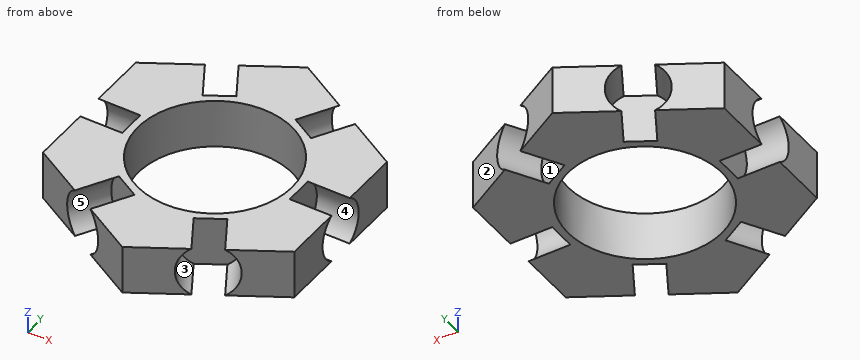
from build123d import *

# Parameters (mm, degrees)
SKETCH1_R           = 11
BOSS_EXTRUDE1_DEPTH = 3.5
SKETCH2_R           = 4.05
CUT_EXTRUDE3_DEPTH  = 6
CIRPATTERN1_COUNT   = 6


with BuildPart() as part:
    # Sketch1 → Boss-Extrude1 (new body, symmetric)
    with BuildSketch(Plane.XY):
        Polygon((18, -10.392304845), (18, 10.392304845), (0, 20.784609691), (-18, 10.392304845), (-18, -10.392304845), (0, -20.784609691), align=None)
        Circle(SKETCH1_R, mode=Mode.SUBTRACT)
    extrude(amount=BOSS_EXTRUDE1_DEPTH, both=True)

    # Sketch2 → Cut-Extrude3 (cut)
    with BuildSketch(Plane(origin=(-12.610372246, -13.50400788, 0), x_dir=(0.866025404, -0.5, 0), z_dir=(0.5, 0.866025404, 0))):
        with Locations((4.168898776, 0)):
            Circle(SKETCH2_R)
    cut_extrude3 = extrude(amount=CUT_EXTRUDE3_DEPTH, mode=Mode.SUBTRACT)

    # CirPattern1: Cut-Extrude3 ×6 about axis
    cirpattern1_axis = Axis((0, 0, 0), (0, 0, 1))
    for i in range(1, CIRPATTERN1_COUNT):
        add(cut_extrude3.rotate(cirpattern1_axis, i * 360 / CIRPATTERN1_COUNT), mode=Mode.SUBTRACT)


solid = part.part
CAD build for the part. Positions are in the model's coordinates, mm. Face numbers are marked on the shaded views. A direction names the side the tool comes from. Give positions to 0.01 mm unless a question says otherwise; leave off trailing zeros. Write each loop counter-clockwise with the first axis right and the second up, starting at its lowest first coordinate (ties: lowest second). Pieces come first, ordered by that corner, then holes. Notation, with made-up numbers: (-17.5, 87.25) - (25.5, 87.25) arc R24 cw to (25.5, 107.25) - close; hole circle Ø9 at (26.5, 81.5). An arc over 180 degrees is marked (long way). Put each result on its own line as item: value.
(1) Saw through at A-A (y = 0). List the corners of the cut face in (x, z), then the cut area to 3 significant figures.
Working result:
outline: (-12, -3.5) - (-11, -3.5) - (-11, 3.5) - (-12, 3.5) - close; (11, -3.5) - (12, -3.5) - (12, 3.5) - (11, 3.5) - close
area: 14.0 mm^2
(2) Wall check: L1, parallel to Y at x = 0, z = 0.5; L2, parallel to X at y = 10, z = -3; L3, parallel to X at y = 9, z = 1.5. Give the ranges that are in metal, low to high.
Working result:
L1: -20.78 to -11, 11 to 20.78
L2: -18 to -8.92, -6.68 to -4.58, 4.58 to 6.68, 8.92 to 18
L3: -18 to -9.54, -8.41 to -6.32, 6.32 to 8.41, 9.54 to 18
(3) Drop a flat-ended pin along its axis: pin 1 Ø2 at (y, z) = (-0.5, -1.5) entering from +X. Give the stop position or say it passes through.
Working result:
pin 1: x = 12
(4) Pull direction Z, two halves, no side cores. Call the marked faces 1 and 2: released by +Z, released by -Z, zero draft, split by the parting line, or undercut.
Working result:
face 1: undercut
face 2: zero draft
(5) Saw through at C-C (x = -5.5). Count the separate pieces of the cut face and the enclosed holes in it, then the cut area to 3 significant figures.
Working result:
separate pieces: 6
enclosed holes: 0
area: 32.3 mm^2
(6) Tool access for the marked faces 3, 4 and 5: list every direction of +Z, -Z, +X, -X, +Y, -Y with a clear straight run to the whole face (end or side of a thin tool).
Working result:
face 3: none
face 4: +X
face 5: -Y
